Could you check a few things on this drawing? It's one solid part, dimensions in mm from its lowest x, y, z. A direction names the side the tool comes from. Round coordinates to 2 decimals unless told otherwise and drop trailing zeros. Loops run counter-clockwise (first coordinate to the right, second up) from the corner with the lowest first, then second, coordinate; pieces in that order, holes last. Notation, with made-up numbers: M -4,33.5 L 4,33.5 A33 ccw 4,70.5 Z; hole C 86,3.25 d9. An arc over 180 degrees is marked long. Answer as a JSON object with one key per item and string values.
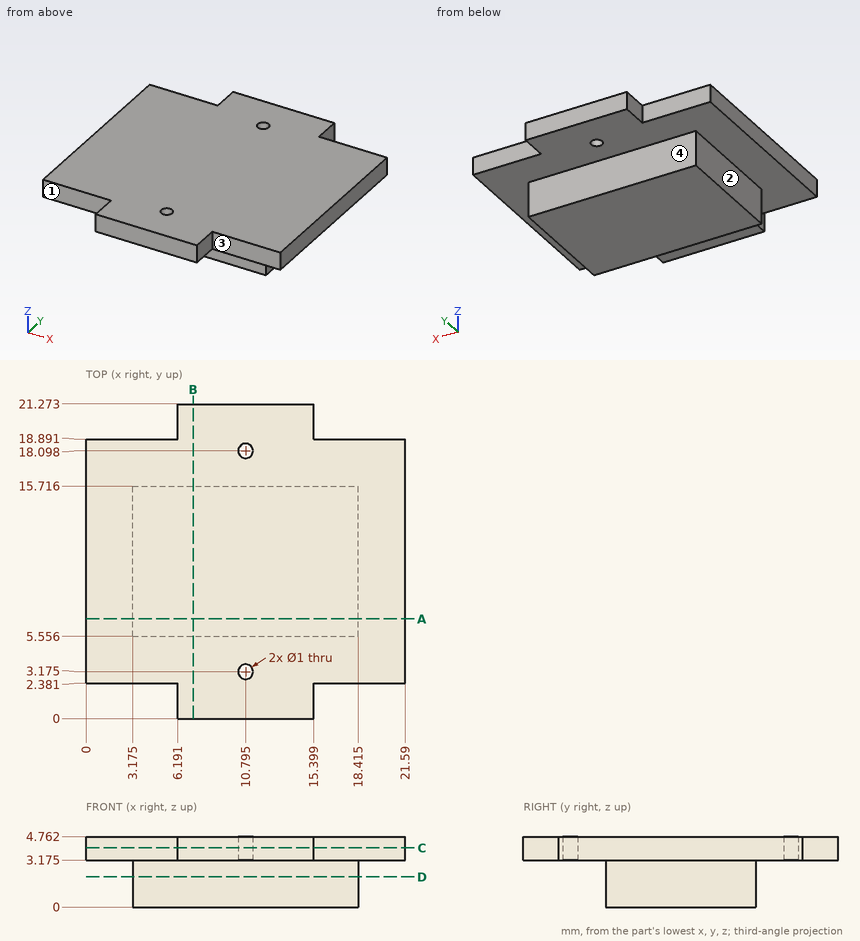
Item 1: I want a section at C-C, the plane z = 4. Please give me the cut outline in (x, y) (1 decimal), then the cut area to 3 significant figures.
Resolved:
{"outline": "M 0,2.4 L 6.2,2.4 L 6.2,0 L 15.4,0 L 15.4,2.4 L 21.6,2.4 L 21.6,18.9 L 15.4,18.9 L 15.4,21.3 L 6.2,21.3 L 6.2,18.9 L 0,18.9 Z; hole C 10.8,3.2 d1; hole C 10.8,18.1 d1", "area": "399 mm²"}
Item 2: I want a section at B-B, the plane x = 7.25. Please give me the cut outline in (y, z) (1 decimal).
Resolved:
{"outline": "M 0,3.2 L 5.6,3.2 L 5.6,0 L 15.7,0 L 15.7,3.2 L 21.3,3.2 L 21.3,4.8 L 0,4.8 Z"}
Item 3: On a 3-axis mill with a long thin cutter (end or side, diameter ignored), from which of +Z, -Z, +X, -X, +Y, -Y can I reach the whole of each face in a straight line? I mean the marked faces 1, 2, 3 and 4. Say none if no direction works.
Resolved:
{"face 1": "+Z, -Z, -X, -Y", "face 2": "-Z, -X, +Y, -Y", "face 3": "+Z, -Z, +X, -Y", "face 4": "-Z, +X, -X, +Y"}
Item 4: Please list where these lines run through material, in increasing order: probe 1 along X at (y, z) = (12.25, 2.2) (1 decimal); probe 2 along Y at (x, z) = (16.25, 0.25); probe 3 along Z at (x, y) = (10.25, 3) (1 decimal). Write a range as from..to.
Resolved:
{"probe 1": "3.2..18.4", "probe 2": "5.56..15.72", "probe 3": "3.2..4.8"}
Item 5: I'm going to push flat-ended pins straight in: pin 1 Ø0.5 at (x, z) = (18.5, 4) entering from +Y; pin 2 Ø0.8 at (y, z) = (1.5, 4) entering from -X; pin 3 Ø1 at (y, z) = (12.5, 1) entering from -X (1 decimal). Where does each tip first touch, or does it pass through?
Resolved:
{"pin 1": "y = 18.89", "pin 2": "x = 6.19", "pin 3": "x = 3.2"}
Item 6: I want a section at D-D, the plane z = 2.05. Please give me the cut outline in (x, y) (1 decimal), then the cut area to 3 significant figures.
Resolved:
{"outline": "M 3.2,5.6 L 18.4,5.6 L 18.4,15.7 L 3.2,15.7 Z", "area": "155 mm²"}
Item 7: I want a section at A-A, the plane y = 6.75. Please give me the cut outline in (x, z) (1 decimal).
Resolved:
{"outline": "M 0,3.2 L 3.2,3.2 L 3.2,0 L 18.4,0 L 18.4,3.2 L 21.6,3.2 L 21.6,4.8 L 0,4.8 Z"}
